from build123d import *

# Parameters (mm, degrees)
EXTRUDE1_DEPTH     = 100
EXTRUDE5_DEPTH     = 3
SKETCH17_W         = 35
SKETCH17_H         = 13.283913387
CUT_EXTRUDE1_DEPTH = 100
SKETCH19_W         = 24.898249574
SKETCH19_H         = 2.5
CUT_EXTRUDE2_DEPTH = 100
CUT_EXTRUDE3_DEPTH = 98
SKETCH21_W         = 6.656858378
SKETCH21_H         = 5.544933951
CUT_EXTRUDE5_DEPTH = 3
SKETCH23_W         = 11.264163756
SKETCH23_H         = 3.071962193
CUT_EXTRUDE6_DEPTH = 3
SKETCH24_W         = 6.656858378
SKETCH24_H         = 5.544933951
CUT_EXTRUDE7_DEPTH = 3
SKETCH25_W         = 8.129030682
SKETCH25_H         = 5.409731787
CUT_EXTRUDE8_DEPTH = 3


with BuildPart() as part:
    # Sketch1 → Extrude1 (new body)
    with BuildSketch(Plane.XY):
        with BuildLine():
            Line((24.434543456, 1.743114855), (35, 24.400809531))
            ThreePointArc((35, 24.400809531), (20.23335986, 8.279731765), (0, 0))
            Line((0, 0), (4.510649495, 0))
            Line((4.510649495, 0), (24.434543456, 1.743114855))
        make_face()
    extrude(amount=EXTRUDE1_DEPTH)

    # Sketch10 → Extrude5 (cut)
    with BuildSketch(Plane.XY.offset(100)):
        Polygon((27.084425545, 11.426798952), (29.084425545, 11.066694717), (24.434543456, 1.743114855), (17.054195147, 3.071962193), align=None)
    extrude5 = extrude(amount=-EXTRUDE5_DEPTH, mode=Mode.SUBTRACT)

    # Mirror2: Extrude5 across plane
    add(extrude5.mirror(Plane.XY.offset(50)), mode=Mode.SUBTRACT)

    # Sketch16 → M2.5 Clearance Hole2 (revolve, cut)
    with BuildSketch(Plane(origin=(24.120076457, 5.864055695, 97), x_dir=(0, -1, 0), z_dir=(1, 0, 0))):
        Polygon((0, 0), (0, 16.871247898), (1.45, 16), (1.45, 0), align=None)
    m2_5_clearance_hole2 = revolve(axis=Axis((24.120076457, 5.864055695, 103.35), (0, 0, -1)), mode=Mode.SUBTRACT)

    # Mirror3: M2.5 Clearance Hole2 across plane
    add(m2_5_clearance_hole2.mirror(Plane.XY.offset(50)), mode=Mode.SUBTRACT)

    # Sketch17 → Cut-Extrude1 (cut)
    with BuildSketch(Plane.XY.offset(100)):
        with Locations((17.5, 17.758852838)):
            Rectangle(SKETCH17_W, SKETCH17_H)
    extrude(amount=-CUT_EXTRUDE1_DEPTH, mode=Mode.SUBTRACT)

    # Sketch19 → Cut-Extrude2 (cut)
    with BuildSketch(Plane.XY.offset(100)):
        with Locations((16.356484671, 9.866896144)):
            Rectangle(SKETCH19_W, SKETCH19_H)
    extrude(amount=-CUT_EXTRUDE2_DEPTH, mode=Mode.SUBTRACT)

    # Sketch20 → Cut-Extrude3 (cut)
    with BuildSketch(Plane.XY.offset(100)):
        Polygon((6.18702488, 0.620277991), (15.948528927, 4.330532923), (15.948528927, 1.543663509), align=None)
    extrude(amount=-CUT_EXTRUDE3_DEPTH, mode=Mode.SUBTRACT)

    # Sketch21 → Cut-Extrude5 (cut)
    with BuildSketch(Plane.XY.offset(100)):
        with Locations((20.382624336, 5.844429168)):
            Rectangle(SKETCH21_W, SKETCH21_H)
    extrude(amount=-CUT_EXTRUDE5_DEPTH, mode=Mode.SUBTRACT)

    # Sketch23 → Cut-Extrude6 (cut)
    with BuildSketch(Plane.XY.offset(100)):
        with Locations((22.686277025, 1.535981097)):
            Rectangle(SKETCH23_W, SKETCH23_H)
    extrude(amount=-CUT_EXTRUDE6_DEPTH, mode=Mode.SUBTRACT)

    # Sketch24 → Cut-Extrude7 (cut)
    with BuildSketch(Plane(origin=(0, 0, 0), x_dir=(-1, 0, 0), z_dir=(0, 0, -1))):
        with Locations((-20.382624336, 5.844429168)):
            Rectangle(SKETCH24_W, SKETCH24_H)
    extrude(amount=-CUT_EXTRUDE7_DEPTH, mode=Mode.SUBTRACT)

    # Sketch25 → Cut-Extrude8 (cut)
    with BuildSketch(Plane(origin=(0, 0, 0), x_dir=(-1, 0, 0), z_dir=(0, 0, -1))):
        with Locations((-21.118710488, 0.3670963)):
            Rectangle(SKETCH25_W, SKETCH25_H)
    extrude(amount=-CUT_EXTRUDE8_DEPTH, mode=Mode.SUBTRACT)


solid = part.part
The model under review builds one solid part; all positions refer to its coordinate system, in mm. A direction names the side the tool comes from. Coordinates: 2 decimals unless noted, no trailing zeros. Loops run counter-clockwise (first coordinate to the right, second up) from the corner with the lowest first, then second, coordinate; pieces in that order, holes last.
(1) Consider section B-B, the plane x = 13.75. Give the boundary of the cut face in (y, z).
Determined:
outline: (0.81, 0) - (4.45, 0) - (4.45, 100) - (3.49, 100) - (3.49, 2) - (1.34, 2) - (1.34, 100) - (0.81, 100) - close
(2) Tool access review of faces 1 (the flat face through (15.949, 3, 52)), 2 (the flat face through (24, 8.617, 51)), 3 (the cylindrical face through (25.536, 6.178, 10.888)), 4 (the flat face through (17.054, 4, 99)), 5 (the flat face through (21, 5, 3)): name each direction out of +Z, -Z, +X, -X, +Y, -Y from which nothing blocks a thin tool from reaching the whole face with its end or side.
Determined:
face 1: +Z
face 2: +Z, -Z, +X, -X, +Y
face 3: -Z
face 4: +Z, +X, +Y, -Y
face 5: -Z, +X, +Y, -Y
(3) Consider section C-C, the plane z = 86.5. Give the boundary of the cut face in (x, y).
Determined:
outline: (0, 0) - (4.51, 0) - (24.43, 1.74) - (27.64, 8.62) - (20.71, 8.62) arc R50 cw to start; hole (6.19, 0.62) - (15.95, 1.54) - (15.95, 4.33) - close; hole circle Ø2.9 at (24.12, 5.86)
(4) Insertion check: P1, Ø5, axis at x = 11.5, y = 6.5, coming from the -Z side; P2, Ø3, axis at x = 17, z = 44.5, coming from the +Y side; P3, Ø2.5, axis at x = 24.12, y = 5.86, coming from the +Z side; P4, Ø4, axis at x = 20, y = 6, coming from the +Z side. Each pin has a flat end and moves straight along its axis. Give the tip position at first contact, or say it passes through.
Determined:
P1: passes through
P2: stops at y = 7.12
P3: stops at z = 80.88
P4: stops at z = 97
(5) Draft analysis for pull direction Y (two halves, no side actions). For faces 6 (the cylindrical face through (25.536, 6.178, 89.112)), 7 (the flat face through (17.054, 4, 1)), 8 (the flat face through (14.33, 0.86, 49.3)), state which applies: +Y half, -Y half, draft (parallel to the pull), parting line (faces both ways), or undercut.
Determined:
face 6: undercut
face 7: draft
face 8: -Y half
(6) Consider section A-A, the plane z = 34. Give the boundary of the cut face in (x, y), plus the area to 3 significant figures.
Determined:
outline: (0, 0) - (4.51, 0) - (24.43, 1.74) - (27.64, 8.62) - (20.71, 8.62) arc R50 cw to start; hole (6.19, 0.62) - (15.95, 1.54) - (15.95, 4.33) - close
area: 82.3 mm2
(7) Wall thickness on L1, parallel to Y at x = 13, z = 43; L2, parallel to Z at x = 18.5, y = 6.75; L3, parallel to Y at x = 22, z = 83: over which ranges is each line inside the solid? List them lowest first.
Determined:
L1: y = 0.74 to 1.26, 3.21 to 4.09
L2: z = 3 to 97
L3: y = 1.53 to 8.62
